Work out the finished part from the listing and answer in its coordinate system (mm). Coordinates: 2 decimals unless noted, no trailing zeros. Loops run counter-clockwise (first coordinate to the right, second up) from the corner with the lowest first, then second, coordinate; pieces in that order, holes last.
```python
from build123d import *

# Parameters (mm, degrees)
ESBO_O1_R                = 4.25
RESSALTO_EXTRUS_O1_DEPTH = 3
ESBO_O2_W                = 150
ESBO_O2_H                = 38.52
RESSALTO_EXTRUS_O2_DEPTH = 5
RESSALTO_EXTRUS_O3_START = -25
RESSALTO_EXTRUS_O3_DEPTH = 100
ESBO_O4_R                = 1.75
CORTE_EXTRUS_O1_DEPTH    = 10


with BuildPart() as part:
    # Esboço1 → Ressalto-extrusão1 (new body)
    with BuildSketch(Plane.XY):
        with BuildLine():
            Line((-85.207100592, 26.183431953), (64.792899408, 26.183431953))
            ThreePointArc((64.792899408, 26.183431953), (79.792899408, 11.183431953), (64.792899408, -3.816568047))
            Line((64.792899408, -3.816568047), (-85.207100592, -3.816568047))
            ThreePointArc((-85.207100592, -3.816568047), (-100.207100592, 11.183431953), (-85.207100592, 26.183431953))
        make_face()
        with Locations((-85.207100592, 11.183431953)):
            Circle(ESBO_O1_R, mode=Mode.SUBTRACT)
        with Locations((64.792899408, 11.183431953)):
            Circle(ESBO_O1_R, mode=Mode.SUBTRACT)
    extrude(amount=RESSALTO_EXTRUS_O1_DEPTH)

    # Esboço2 → Ressalto-extrusão2 (add)
    with BuildSketch(Plane(origin=(0, 26.183431953, 0), x_dir=(1, 0, 0), z_dir=(0, 1, 0))):
        with Locations((-10.207100592, -1.5)):
            Rectangle(ESBO_O2_W, ESBO_O2_H)
    extrude(amount=RESSALTO_EXTRUS_O2_DEPTH)

    # Esboço3 → Ressalto-extrusão3 (add)
    with BuildSketch(Plane.ZY.offset(85.207100592).offset(RESSALTO_EXTRUS_O3_START)):
        Polygon((3, 19.683431953), (9.5, 26.183431953), (3, 26.183431953), align=None)
        Polygon((0, 26.183431953), (0, 19.683431953), (-6.5, 26.183431953), align=None)
    extrude(amount=-RESSALTO_EXTRUS_O3_DEPTH)

    # Esboço4 → Corte-extrusão1 (cut)
    with BuildSketch(Plane(origin=(0, 31.183431953, 0), x_dir=(1, 0, 0), z_dir=(0, 1, 0))):
        with Locations(Location((17.512899408, 10.26, 0), (0, 0, 270))):
            Circle(ESBO_O4_R)
        with Locations(Location((17.512899408, -13.26, 0), (0, 0, 270))):
            Circle(ESBO_O4_R)
        with Locations(Location((-57.927100592, -13.26, 0), (0, 0, 270))):
            Circle(ESBO_O4_R)
        with Locations(Location((-57.927100592, 10.26, 0), (0, 0, 270))):
            Circle(ESBO_O4_R)
    extrude(amount=-CORTE_EXTRUS_O1_DEPTH, mode=Mode.SUBTRACT)


solid = part.part
```
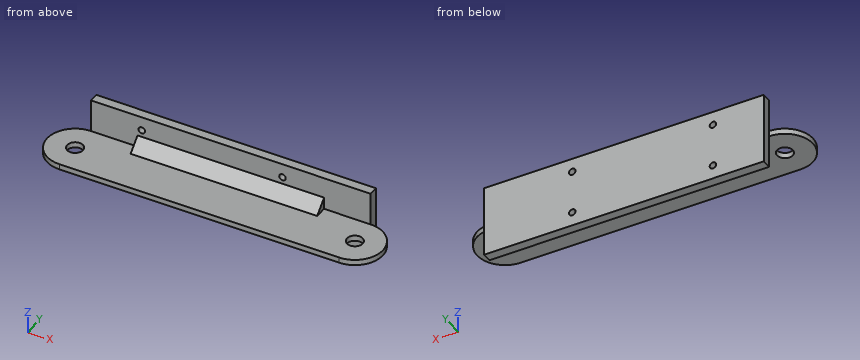
1. A cutting plane is placed at B-B, the plane x = 51.5. Give the vertices of the cut face in (y, z), then the cut area to 3 significant figures.
2. A cutting plane is placed at D-D, the plane y = 22.5. Give the vertices of the cut face in (x, z).
3. Each of these flat-tipped pins is pushed along its axis until it touches: P1, Ø2, axis at y = 23, z = -3, coming from the +X side; P2, Ø5, axis at y = 27.5, z = 7, coming from the +X side; P3, Ø2, axis at y = 22, z = -1.5, coming from the -X side; P4, Ø1, axis at y = 20, z = 6, coming from the +X side. Where does it stop, or does it pass through?
4. Straight lines are drawn through the part: probe 1 along X at (y, z) = (28.1, 13.26); probe 2 along Z at (x, y) = (52.5, 11.5); probe 3 along Y at (x, z) = (-3.5, -13.5). For each, find the intervals that lie inside material, in ascending order.
5. A cutting plane is placed at C-C, the plane y = 13. Give the vertices of the cut face in (x, z), then the cut area to 3 significant figures.
6. A cutting plane is placed at A-A, the plane z = -10.26. Give the vertices of the cut face in (x, y).
Answers below:
1. outline: (-3.82, 0) - (26.18, 0) - (26.18, -17.76) - (31.18, -17.76) - (31.18, 20.76) - (26.18, 20.76) - (26.18, 3) - (-3.82, 3) - close
1. area: 283 mm2
2. outline: (-95.05, 0) - (-60.21, 0) - (-60.21, -2.82) - (39.79, -2.82) - (39.79, 0) - (74.64, 0) - (74.64, 3) - (39.79, 3) - (39.79, 5.82) - (-60.21, 5.82) - (-60.21, 3) - (-95.05, 3) - close
3. P1: stops at x = 39.79
3. P2: stops at x = 64.79
3. P3: stops at x = -60.21
3. P4: passes through
4. probe 1: x = -85.21 to -59.68, -56.18 to 15.76, 19.26 to 64.79
4. probe 2: z = 0 to 3
4. probe 3: y = 26.18 to 31.18
5. outline: (-100.1, 0) - (-89.05, 0) - (-89.05, 3) - (-100.1, 3) - close; (-81.36, 0) - (60.95, 0) - (60.95, 3) - (-81.36, 3) - close; (68.64, 0) - (79.68, 0) - (79.68, 3) - (68.64, 3) - close
5. area: 493 mm2
6. outline: (-85.21, 26.18) - (-59.68, 26.18) - (-59.68, 31.18) - (-85.21, 31.18) - close; (-56.18, 26.18) - (15.76, 26.18) - (15.76, 31.18) - (-56.18, 31.18) - close; (19.26, 26.18) - (64.79, 26.18) - (64.79, 31.18) - (19.26, 31.18) - close
